from build123d import *

# Parameters (mm, degrees)
SKETCH_1_W      = 90
SKETCH_1_H      = 45
EXTRUDE_1_DEPTH = 3
SKETCH_2_R      = 2.5
DIA_5_DEPTH     = 101.667770413
SKETCH_3_R      = 1.5
DIA_3_DEPTH     = 101.667770413


with BuildPart() as part:
    # 草圖1 → 伸長1 (new body)
    with BuildSketch(Plane.XY):
        with Locations((45, 22.5)):
            Rectangle(SKETCH_1_W, SKETCH_1_H)
    extrude(amount=EXTRUDE_1_DEPTH)

    # 草圖2 → Dia 5 (cut, through all)
    with BuildSketch(Plane.XY.offset(3)):
        with Locations((6, 38)):
            Circle(SKETCH_2_R)
    extrude(amount=-DIA_5_DEPTH, mode=Mode.SUBTRACT)

    # 草圖3 → Dia 3 (cut, through all)
    with BuildSketch(Plane.XY.offset(3)):
        with Locations((16, 38)):
            Circle(SKETCH_3_R)
    extrude(amount=-DIA_3_DEPTH, mode=Mode.SUBTRACT)


solid = part.part
Geometry: final body of the model. Coordinates: model frame, mm. Round coordinates to 2 decimals unless told otherwise and drop trailing zeros. Loops run counter-clockwise (first coordinate to the right, second up) from the corner with the lowest first, then second, coordinate; pieces in that order, holes last. Notation, with made-up numbers: (54.5, 14.5) -> (105.5, 14.5) arc R29 cw to (105.5, 40.5) -> close; hole circle Ø11 at (2.5, 66.5). An arc over 180 degrees is marked (long way). One line per question, with ' | ' between items. Start each with the question number.
1. Mould query, pull axis Y, two halves, no side actions, for faces 1 (the face through (44, 0, 1)), 2 (the face through (44, 23, 0)), 3 (the face through (14.8, 37.1, 1.5)). Classes: pulls with the +Y half, pulls with the -Y half, needs draft (parallel to the pull), parting line crosses it, or undercut.
2. Line query: line 1 along Y through (x, z) = (6, 0.8); line 2 along Y through (x, z) = (16, 0.6); line 3 along X through (y, z) = (39, 0.1). Output: solid intervals per line, ascending. Write a range as [from, to].
3. Section A-A on x = 6. Output: boundary loops of the cut face in (y, z), and give its area (3 significant figures).
4. Section C-C on x = 16. Output: boundary loops of the cut face in (y, z).
5. Section B-B on y = 38. Output: boundary loops of the cut face in (x, z), and give its area (3 significant figures).
Returned:
1) face 1: pulls with the -Y half | face 2: needs draft | face 3: undercut
2) line 1: y = [0, 35.5], [40.5, 45] | line 2: y = [0, 36.5], [39.5, 45] | line 3: x = [0, 3.71], [8.29, 14.88], [17.12, 90]
3) outline: (0, 0) -> (35.5, 0) -> (35.5, 3) -> (0, 3) -> close; (40.5, 0) -> (45, 0) -> (45, 3) -> (40.5, 3) -> close | area: 120 mm2
4) outline: (0, 0) -> (36.5, 0) -> (36.5, 3) -> (0, 3) -> close; (39.5, 0) -> (45, 0) -> (45, 3) -> (39.5, 3) -> close
5) outline: (0, 0) -> (3.5, 0) -> (3.5, 3) -> (0, 3) -> close; (8.5, 0) -> (14.5, 0) -> (14.5, 3) -> (8.5, 3) -> close; (17.5, 0) -> (90, 0) -> (90, 3) -> (17.5, 3) -> close | area: 246 mm2
